```python
from build123d import *

# Parameters (mm, degrees)
EXTRUDE_1_DEPTH      = 6
EXTRUDE_1_DEPTH_BACK = 6
SKETCH_1_R           = 4
SKETCH_2_R           = 7
CUT_EXTRUDE_1_DEPTH  = 2
CUT_EXTRUDE_START    = -2
SKETCH_3_R           = 7
CUT_EXTRUDE_2_DEPTH  = 2
SKETCH_4_R           = 2.75
CUT_EXTRUDE_3_DEPTH  = 17


with BuildPart() as part:
    # Sketch 1 → Extrude 1 (new, two sides: drawn at the far end of the back side and taken through both)
    with BuildSketch(Plane.XY.offset(-EXTRUDE_1_DEPTH_BACK)):
        with BuildLine():
            Line((3.5, 15), (-3.5, 15))
            ThreePointArc((-3.5, 15), (-11.278174593, 11.778174593), (-14.5, 4))
            Line((-14.5, 4), (-14.5, -10))
            Line((-14.5, -10), (-26.5, -10))
            Line((-26.5, -10), (-26.5, -20))
            Line((-26.5, -20), (26.5, -20))
            Line((26.5, -20), (26.5, -10))
            Line((26.5, -10), (14.5, -10))
            Line((14.5, -10), (14.5, 4))
            ThreePointArc((14.5, 4), (11.278174593, 11.778174593), (3.5, 15))
        make_face()
        Circle(SKETCH_1_R, mode=Mode.SUBTRACT)
    extrude(amount=EXTRUDE_1_DEPTH + EXTRUDE_1_DEPTH_BACK)

    # Sketch 2 → Cut-Extrude 1 (cut)
    with BuildSketch(Plane.XY.offset(6)):
        Circle(SKETCH_2_R)
    extrude(amount=-CUT_EXTRUDE_1_DEPTH, mode=Mode.SUBTRACT)

    # Sketch 3 → Cut-Extrude 2 (cut)
    with BuildSketch(Plane(origin=(0, 0, -6), x_dir=(-1, 0, 0), z_dir=(0, 0, -1)).offset(CUT_EXTRUDE_START)):
        with Locations(Location((0, 0, 0), (0, 0, 180))):
            Circle(SKETCH_3_R)
    extrude(amount=CUT_EXTRUDE_2_DEPTH, mode=Mode.SUBTRACT)

    # Sketch 4 → Cut-Extrude 3 (cut)
    with BuildSketch(Plane.XZ.offset(20)):
        with Locations(Location((-20.5, 0, 0), (0, 0, 270))):
            Circle(SKETCH_4_R)
        with Locations(Location((20.5, 0, 0), (0, 0, 180))):
            Circle(SKETCH_4_R)
    extrude(amount=-CUT_EXTRUDE_3_DEPTH, mode=Mode.SUBTRACT)


solid = part.part
```
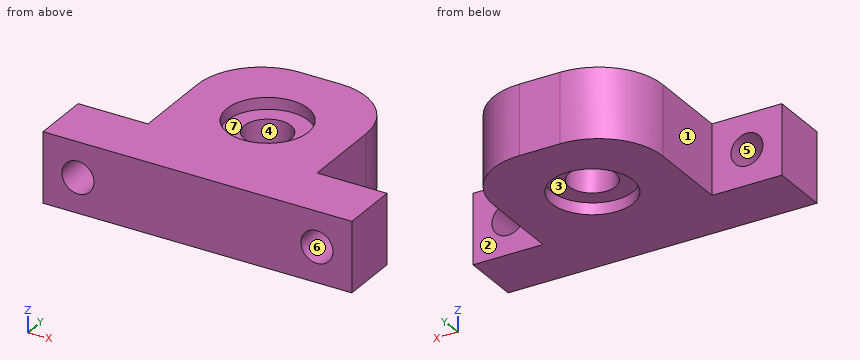
Geometry: final body of the model. Coordinates: model frame, mm. Face numbers are marked on the shaded views. A direction names the side the tool comes from. Coordinates: 2 decimals unless noted, no trailing zeros. Order: outer loops, then holes, each group sorted by start corner. A loop starts at its lowest first (then second) coordinate and runs counter-clockwise, first axis right, second up. Notation, with made-up numbers: (86, 0.25) -> (90, 0.25) arc R5 ccw to (90, 5.25) -> close; hole circle Ø10 at (69.5, -3). An arc over 180 degrees is marked (long way). Write item = value, one per line.
(1) Cut plane D-D on y = 3. Return loops of the section in (x, z), plus the area to 3 significant figures.
Solved:
outline = (-14.5, -6) -> (-6.32, -6) -> (-6.32, -4) -> (-2.65, -4) -> (-2.65, 4) -> (-6.32, 4) -> (-6.32, 6) -> (-14.5, 6) -> close; (2.65, -4) -> (6.32, -4) -> (6.32, -6) -> (14.5, -6) -> (14.5, 6) -> (6.32, 6) -> (6.32, 4) -> (2.65, 4) -> close
area = 255 mm²
(2) Cut plane A-A on z = 0. Return loops of the section in (x, y).
Solved:
outline = (-26.5, -20) -> (-23.25, -20) -> (-23.25, -10) -> (-26.5, -10) -> close; (-17.75, -20) -> (17.75, -20) -> (17.75, -10) -> (14.5, -10) -> (14.5, 4) arc R11 ccw to (3.5, 15) -> (-3.5, 15) arc R11 ccw to (-14.5, 4) -> (-14.5, -10) -> (-17.75, -10) -> close; (23.25, -20) -> (26.5, -20) -> (26.5, -10) -> (23.25, -10) -> close; hole circle Ø8 at (0, 0)
(3) Cut plane C-C on z = -5. Return loops of the section in (x, y), plus the area to 3 significant figures.
Solved:
outline = (-26.5, -20) -> (26.5, -20) -> (26.5, -10) -> (14.5, -10) -> (14.5, 4) arc R11 ccw to (3.5, 15) -> (-3.5, 15) arc R11 ccw to (-14.5, 4) -> (-14.5, -10) -> (-26.5, -10) -> close; hole circle Ø14 at (0, 0)
area = 1,050 mm²
(4) Cut plane B-B on x = 0. Return loops of the section in (y, z).
Solved:
outline = (-20, -6) -> (-7, -6) -> (-7, -4) -> (-4, -4) -> (-4, 4) -> (-7, 4) -> (-7, 6) -> (-20, 6) -> close; (4, -4) -> (7, -4) -> (7, -6) -> (15, -6) -> (15, 6) -> (7, 6) -> (7, 4) -> (4, 4) -> close
(5) Access query for the marked faces 1, 2 and 3. Directions: +Z, -Z, +X, -X, +Y, -Y. A direction counts if a zero-diameter tool reaches every point of the face in a straight line with its end or side. Return the directions, or none.
Solved:
face_1 = +Z, -Z, -X, +Y
face_2 = +Z, -Z, +X, +Y
face_3 = -Z
(6) Pin query (flat end, axial travel): pin 1 Ø3.5 at (x, z) = (18, -1) entering from +Y; pin 2 Ø8.5 at (x, y) = (0, 0) entering from -Z; pin 3 Ø1 at (x, z) = (5.5, -1) entering from +Y. Return the tip coordinate at first contact, or that it passes through.
Solved:
pin_1 = -10
pin_2 = -4
pin_3 = 14.9
(7) Line query: line 1 (Y direction, x = 0, z = -2.25); line 2 (Y direction, x = -16.5, z = 2.5); line 3 (Y direction, x = -1, z = 5). Output: solid intervals per line, ascending.
Solved:
line_1 = -20 to -4, 4 to 15
line_2 = -20 to -10
line_3 = -20 to -6.93, 6.93 to 15
(8) Pull-direction query (Z, two-part tool) for the marked faces 4, 5, 6 and 7; classes: pulls with the +Z half, pulls with the -Z half, needs draft (parallel to the pull), parting line crosses it, or undercut.
Solved:
face_4 = needs draft
face_5 = undercut
face_6 = undercut
face_7 = pulls with the +Z half
